Study the drawing (mm; zero at the part's minimum x, y, z) and answer. Coordinates: 2 decimals unless noted, no trailing zeros. Loops run counter-clockwise (first coordinate to the right, second up) from the corner with the lowest first, then second, coordinate; pieces in that order, holes last. Notation, with made-up numbers: (17, -28.5) -> (40, -28.5) arc R30 ccw to (40, 4.5) -> close; hole circle Ø1 at (-17, -9). An arc over 180 degrees is marked (long way). Answer in a Markdown table with one row per item.
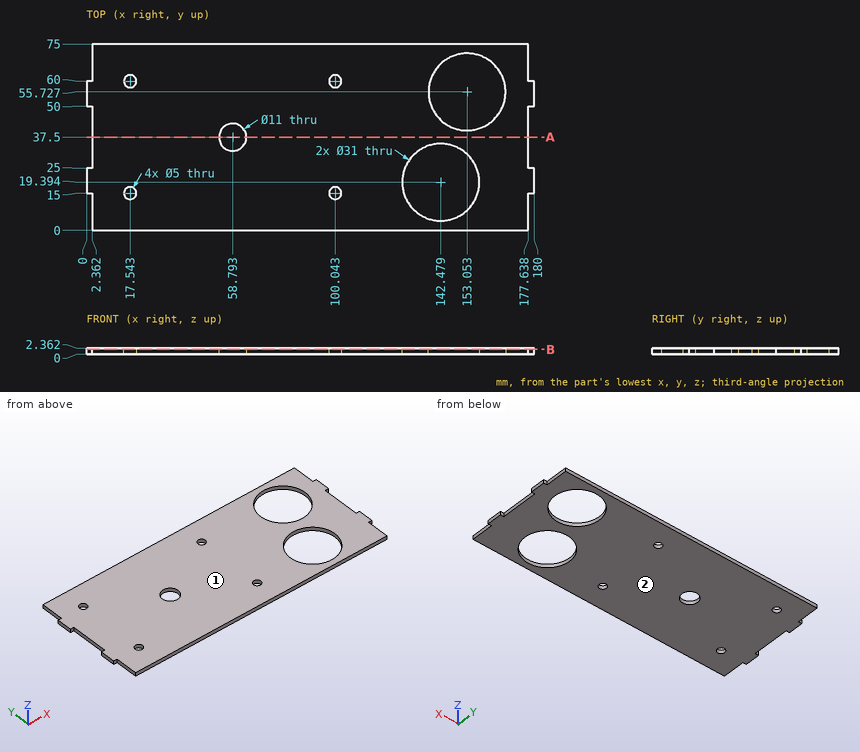
1. A cutting plane is placed at B-B on z = 2. Give the vertices of the cut face in (x, y) (1 decimal), and give its area (3 significant figures).
A:
| item | result |
|---|---|
| outline | (0, 15) -> (2.4, 15) -> (2.4, 0) -> (177.6, 0) -> (177.6, 15) -> (180, 15) -> (180, 25) -> (177.6, 25) -> (177.6, 50) -> (180, 50) -> (180, 60) -> (177.6, 60) -> (177.6, 75) -> (2.4, 75) -> (2.4, 60) -> (0, 60) -> (0, 50) -> (2.4, 50) -> (2.4, 25) -> (0, 25) -> close; hole circle Ø5 at (17.5, 15); hole circle Ø5 at (17.5, 60); hole circle Ø11 at (58.8, 37.5); hole circle Ø5 at (100, 15); hole circle Ø5 at (100, 60); hole circle Ø31 at (142.5, 19.4); hole circle Ø31 at (153.1, 55.7) |
| area | 11,600 mm2 |
2. A cutting plane is placed at A-A on y = 37.5. Give the vertices of the cut face in (x, z).
A:
| item | result |
|---|---|
| outline | (2.36, 0) -> (53.29, 0) -> (53.29, 2.36) -> (2.36, 2.36) -> close; (64.29, 0) -> (177.64, 0) -> (177.64, 2.36) -> (64.29, 2.36) -> close |
3. The mould has two halves that part along Z. Classify the marked faces 1 and 2: pulls with the +Z half, pulls with the -Z half, needs draft (parallel to the pull), parting line crosses it, or undercut.
A:
| item | result |
|---|---|
| face 1 | pulls with the +Z half |
| face 2 | pulls with the -Z half |
4. Find the intervals of material crossed by probe 1 along X at (y, z) = (60.5, 1.75) (1 decimal); probe 2 along X at (y, z) = (13, 1.7) (1 decimal); probe 3 along Y at (x, z) = (19, 1.45), in increasing order.
A:
| item | result |
|---|---|
| probe 1 | x = 2.4 to 15.1, 20 to 97.6, 102.5 to 138.3, 167.8 to 177.6 |
| probe 2 | x = 2.4 to 16, 19 to 98.5, 101.5 to 128.4, 156.6 to 177.6 |
| probe 3 | y = 0 to 12.97, 17.03 to 57.97, 62.03 to 75 |
5. Given pin 1 Ø6.5 at (x, y) = (17.54, 15) entering from +Z; pin 2 Ø0.7 at (x, z) = (1, 1.5) entering from +Y; pin 3 Ø1.2 at (y, z) = (64.5, 1.5) entering from +X; pin 4 Ø1.2 at (x, z) = (1, 1) entering from -Y, each flat-ended and moving along its own axis, determine where each tip first touches the part or whether it passes through.
A:
| item | result |
|---|---|
| pin 1 | stops at z = 2.36 |
| pin 2 | stops at y = 60 |
| pin 3 | stops at x = 177.64 |
| pin 4 | stops at y = 15 |
